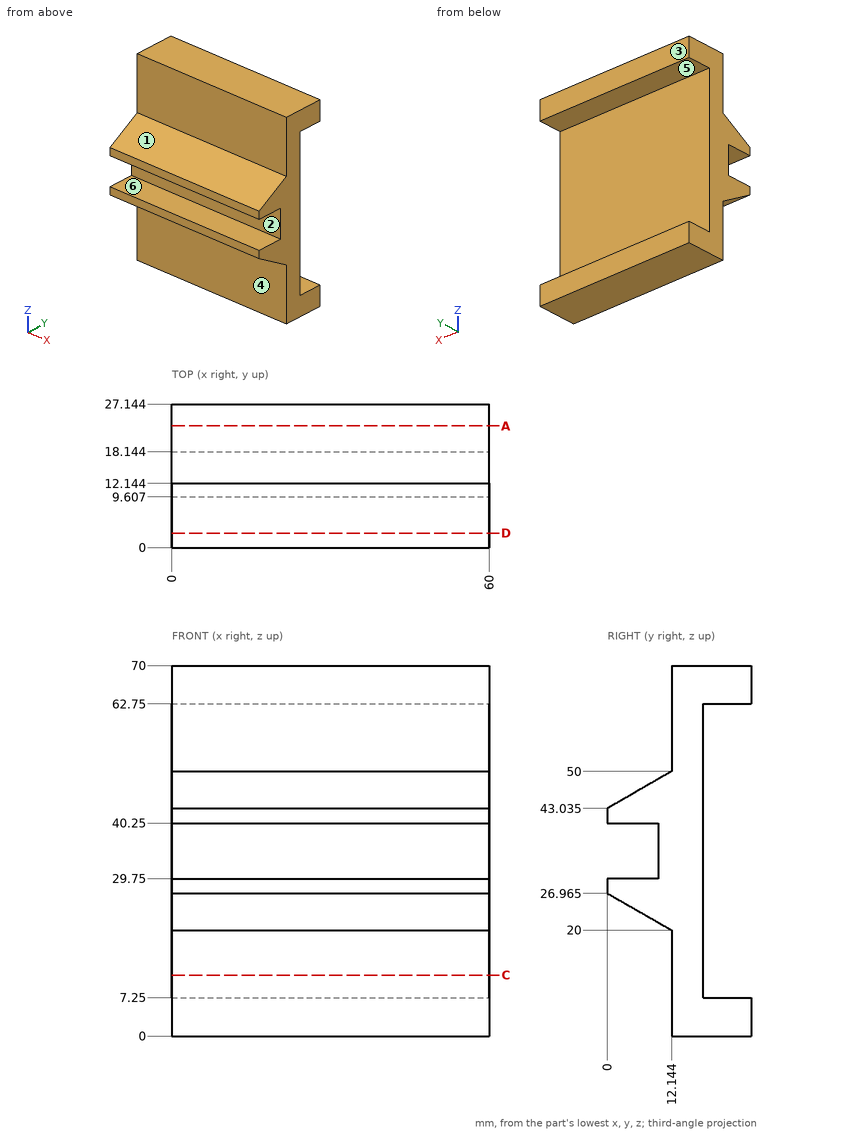
Can you work these out from the drawing? Everything is in mm from the part's minimum corner. A direction names the side the tool comes from. Give positions to 0.01 mm unless a question says otherwise; leave off trailing zeros. Order: outer loops, then holes, each group sorted by start corner. A loop starts at its lowest first (then second) coordinate and runs counter-clockwise, first axis right, second up. Notation, with made-up numbers: M 2,62.25 L 24,62.25 A15 ccw 24,78.25 Z; hole C -6,54.25 d9. An arc over 180 degrees is marked long. Use a Markdown table: item, result. Add a question column.
Item 1: Suppose I cut it at A-A (y = 23). List the corners of the cut face in (x, z) for me.
Item 2: For the marked faces 4, 5 and 6, which set-ups out of +Z, -Z, +X, -X, +Y, -Y let a thin tool reach every point of the face, with its end or its side?
Item 3: We'd pull the mould along Z, two halves only. Please class the marked faces 1, 2 and 3: +Z half, -Z half, draft (parallel to the pull), parting line (faces both ways), or undercut.
Item 4: Suppose I cut it at D-D (y = 2.75). List the corners of the cut face in (x, z) for me.
Item 5: Suppose I cut it at C-C (z = 11.5). List the corners of the cut face in (x, y) for me (1 decimal).
Item 6: Will these pins go through, and if not, where does the flat tip stop? pin 1 (1.5 mm diameter, centred on x = 16.5, z = 18, fed in from +Y) (1 decimal); pin 2 (16 mm diameter, centred on x = 22.5, z = 57, fed in from -Y); pin 3 (4 mm diameter, centred on x = 37, z = 57, fed in from -Y) (1 decimal).
Item 7: If I drill on L1, parallel to Z at x = 15.5, y = 20; L2, parallel to Z at x = 27, y = 9.25; L3, parallel to Y at x = 28.5, z = 33 (1 decimal), over which ranges is the centre line in solid material (lowest first)? Write a range as [from, to].
Answer sheet:
| question | item | result |
|---|---|---|
| 1 | outline | M 0,0 L 60,0 L 60,7.25 L 0,7.25 Z; M 0,62.75 L 60,62.75 L 60,70 L 0,70 Z |
| 2 | face 4 | -Z, +X, -X, -Y |
| 2 | face 5 | +X, -X, +Y |
| 2 | face 6 | +X, -X, -Y |
| 3 | face 1 | +Z half |
| 3 | face 2 | undercut |
| 3 | face 3 | draft |
| 4 | outline | M 0,25.39 L 60,25.39 L 60,29.75 L 0,29.75 Z; M 0,40.25 L 60,40.25 L 60,44.61 L 0,44.61 Z |
| 5 | outline | M 0,12.1 L 60,12.1 L 60,18.1 L 0,18.1 Z |
| 6 | pin 1 | stops at y = 18.1 |
| 6 | pin 2 | stops at y = 10.4 |
| 6 | pin 3 | stops at y = 12.1 |
| 7 | L1 | z = [0, 7.25], [62.75, 70] |
| 7 | L2 | z = [21.66, 29.75], [40.25, 48.34] |
| 7 | L3 | y = [9.6, 18.1] |
